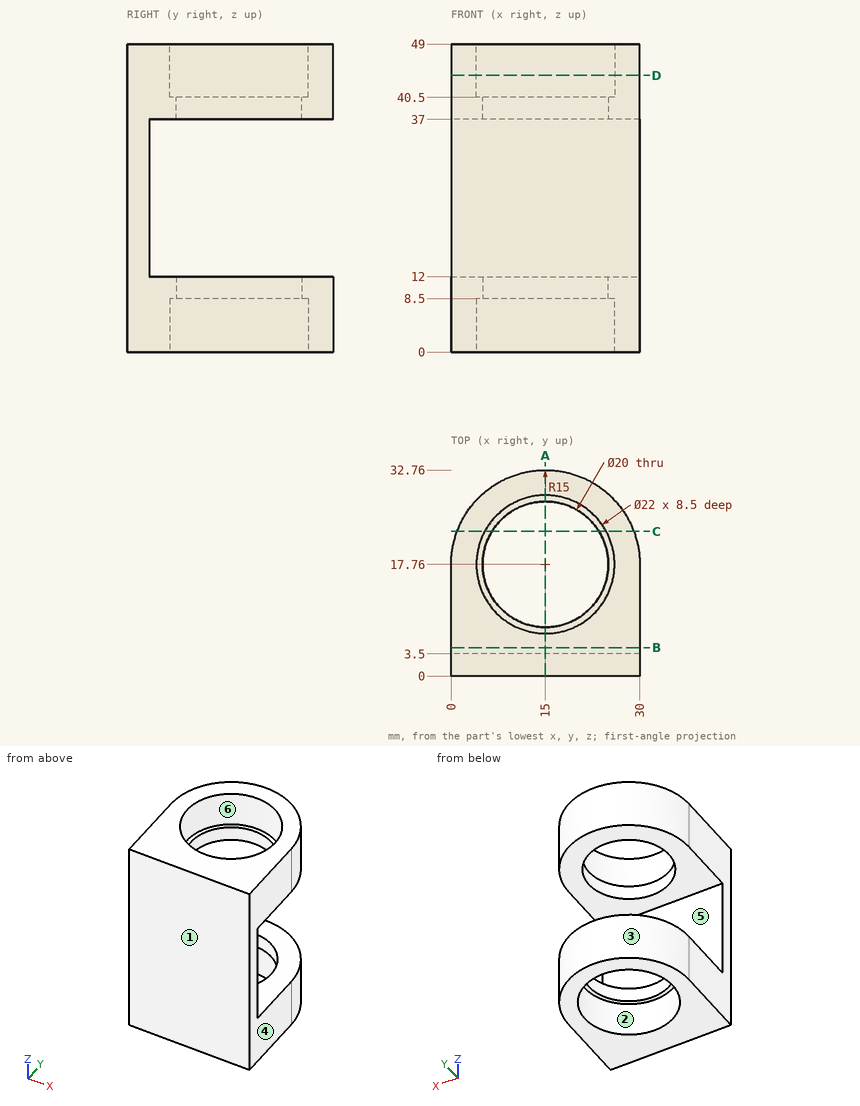
Here's the drawing with two shaded views (mm, measured from the low corner). I have some questions. A direction names the side the tool comes from. Give positions to 0.01 mm unless a question says otherwise; leave off trailing zeros. Order: outer loops, then holes, each group sorted by start corner. A loop starts at its lowest first (then second) coordinate and runs counter-clockwise, first axis right, second up. Notation, with made-up numbers: (-26, -5.5) -> (16, -5.5) arc R37 ccw to (16, 32.5) -> close; hole circle Ø3 at (57, -21). An arc over 180 degrees is marked (long way). One line per item, written item: value. Start each with the question number.
1. Will these pins go through, and if not, where does the flat tip stop? pin 1 Ø9 at (x, y) = (12.5, 15.5) entering from -Z; pin 2 Ø4 at (x, z) = (21.5, 28.5) entering from +Y.
2. We'd pull the mould along X, two halves only. Please class the marked faces 1, 2 and 3: released by +X, released by -X, zero draft, split by the parting line, or undercut.
3. Imagine slicing it at C-C, the plane y = 23. List the corners of the cut face in (x, z) for me.
4. Imagine slicing it at B-B, the plane y = 4.5. List the corners of the cut face in (x, z) for me, plus the area to 3 significant figures.
5. Imagine slicing it at A-A, the plane x = 15. List the corners of the cut face in (y, z) for me.
6. I need wall thicknesses on probe 1 along Z at (x, y) = (5.5, 14); probe 2 along Z at (x, y) = (2.75, 14); probe 3 along Y at (x, z) = (15, 44.5). Which ranges of each line are inside material? Lowest first, please. Write a range as from..to.
7. Imagine slicing it at D-D, the plane z = 44. List the corners of the cut face in (x, y) for me, plus the area to 3 significant figures.
8. For the marked faces 4, 5 and 6, which set-ups out of +Z, -Z, +X, -X, +Y, -Y let a thin tool reach every point of the face, with its end or its side?
Values follow:
1. pin 1: passes through
1. pin 2: stops at y = 3.5
2. face 1: zero draft
2. face 2: undercut
2. face 3: split by the parting line
3. outline: (0.95, 0) -> (5.33, 0) -> (5.33, 8.5) -> (6.48, 8.5) -> (6.48, 12) -> (0.95, 12) -> close; (0.95, 37) -> (6.48, 37) -> (6.48, 40.5) -> (5.33, 40.5) -> (5.33, 49) -> (0.95, 49) -> close; (23.52, 8.5) -> (24.67, 8.5) -> (24.67, 0) -> (29.05, 0) -> (29.05, 12) -> (23.52, 12) -> close; (23.52, 37) -> (29.05, 37) -> (29.05, 49) -> (24.67, 49) -> (24.67, 40.5) -> (23.52, 40.5) -> close
4. outline: (0, 0) -> (30, 0) -> (30, 12) -> (0, 12) -> close; (0, 37) -> (30, 37) -> (30, 49) -> (0, 49) -> close
4. area: 720 mm2
5. outline: (0, 0) -> (6.76, 0) -> (6.76, 8.5) -> (7.76, 8.5) -> (7.76, 12) -> (3.5, 12) -> (3.5, 37) -> (7.76, 37) -> (7.76, 40.5) -> (6.76, 40.5) -> (6.76, 49) -> (0, 49) -> close; (27.76, 8.5) -> (28.76, 8.5) -> (28.76, 0) -> (32.76, 0) -> (32.76, 12) -> (27.76, 12) -> close; (27.76, 37) -> (32.76, 37) -> (32.76, 49) -> (28.76, 49) -> (28.76, 40.5) -> (27.76, 40.5) -> close
6. probe 1: z = 8.5..12, 37..40.5
6. probe 2: z = 0..12, 37..49
6. probe 3: y = 0..6.76, 28.76..32.76
7. outline: (0, 0) -> (30, 0) -> (30, 17.76) arc R15 ccw to (0, 17.76) -> close; hole circle Ø22 at (15, 17.76)
7. area: 506 mm2
8. face 4: +Z, -Z, +X, +Y, -Y
8. face 5: +X, -X, +Y
8. face 6: +Z
